```python
from build123d import *

# Parameters (mm, degrees)
F1_DEPTH = 26.6065


with BuildPart() as f1:
    # F0 (on Right) → F1 (new body, symmetric)
    with BuildSketch(Plane.YZ):
        with BuildLine():
            ThreePointArc((12.446, 2.54), (11.255682, 5.413682), (8.382, 6.604))
            Line((8.382, 6.604), (-8.382, 6.604))
            ThreePointArc((-8.382, 6.604), (-11.255682, 5.413682), (-12.446, 2.54))
            Line((-12.446, 2.54), (-12.446, -6.604))
            Line((-12.446, -6.604), (12.446, -6.604))
            Line((12.446, -6.604), (12.446, 2.54))
        make_face()
    extrude(amount=F1_DEPTH, both=True)


solid = f1.part
```
The listing builds one solid part. Answer for the finished solid, in the listing's coordinates (mm). Coordinates: 2 decimals unless noted, no trailing zeros. Write each loop counter-clockwise with the first axis right and the second up, starting at its lowest first coordinate (ties: lowest second). Pieces come first, ordered by that corner, then holes. Notation, with made-up numbers: (69.25, 32) - (76.25, 32) arc R22 cw to (76.25, 56) - close; hole circle Ø5 at (-38, 46.5). An arc over 180 degrees is marked (long way). Return JSON: item names as keys, results as strings. Group by question number.
Q1. The part is cut by section B-B on y = 9.75. Write down the section's boundary in (x, z).
Q2. Find the intervals of material crossed by line 1 along Y through (x, z) = (3, 4.75); line 2 along Z through (x, y) = (24, 9.75); line 3 along Y through (x, z) = (18.5, 3.25), in increasing order. Write a range as [from, to].
Q3. A flat-ended cylindrical pin translates along its axis: pin 1 Ø1 at (x, z) = (-2, 4) entering from +Y. Find the tip coordinate at first contact, or state that the pin passes through.
Q4. The part is cut by section A-A on x = 17.5. Write down the section's boundary in (y, z), and give its area (3 significant figures).
Evaluation:
{
 "1": {"outline": "(-26.61, -6.6) - (26.61, -6.6) - (26.61, 6.37) - (-26.61, 6.37) - close"},
 "2": {"line 1": "y = [-11.79, 11.79]", "line 2": "z = [-6.6, 6.37]", "line 3": "y = [-12.38, 12.38]"},
 "3": {"pin 1": "stops at y = 12.33"},
 "4": {"outline": "(-12.45, -6.6) - (12.45, -6.6) - (12.45, 2.54) arc R4.06 ccw to (8.38, 6.6) - (-8.38, 6.6) arc R4.06 ccw to (-12.45, 2.54) - close", "area": "322 mm2"}
}
